from build123d import *

# Parameters (mm, degrees)
SKETCH1_W             = 121.412
SKETCH1_H             = 114.4524
BOSS_EXTRUDE1_DEPTH   = 3.175
FILLET2_R             = 13.97
F_6_CLEARANCE_HOLE1_D = 3.7973


with BuildPart() as part:
    # Sketch1 → Boss-Extrude1 (new body)
    with BuildSketch(Plane(origin=(0, 0, 0), x_dir=(1, 0, 0), z_dir=(0, 1, 0))):
        Rectangle(SKETCH1_W, SKETCH1_H)
    extrude(amount=BOSS_EXTRUDE1_DEPTH)

    # Fillet2
    fillet2_edges = [part.edges().sort_by_distance(p)[0] for p in [
        (-60.706, 1.5875, -57.2262),
        (60.706, 1.5875, -57.2262),
        (60.706, 1.5875, 57.2262),
        (-60.706, 1.5875, 57.2262),
    ]]
    fillet(fillet2_edges, radius=FILLET2_R)

    # #6 Clearance Hole1 (through all)
    with Locations(Plane.XZ):
        with Locations((-25.4, 54.0512), (-25.4, -54.0512), (-57.531, -25.4), (-57.531, 25.4)):
            f_6_clearance_hole1 = Hole(F_6_CLEARANCE_HOLE1_D / 2)

    # Mirror1: #6 Clearance Hole1 across plane
    add(f_6_clearance_hole1.mirror(Plane(origin=(0, 0, 0), x_dir=(0, 0, 1), z_dir=(1, 0, 0))), mode=Mode.SUBTRACT)


solid = part.part
CAD build for the part. Positions are in the model's coordinates, mm. Give positions to 0.01 mm unless a question says otherwise; leave off trailing zeros. Write each loop counter-clockwise with the first axis right and the second up, starting at its lowest first coordinate (ties: lowest second). Pieces come first, ordered by that corner, then holes. Notation, with made-up numbers: (-28.75, 24) - (4.25, 24) arc R18 cw to (4.25, 54) - close; hole circle Ø5 at (60, 33.5). An arc over 180 degrees is marked (long way). Put each result on its own line as item: value.
(1) Wall check: L1, parallel to Z at x = 25.4, y = 1.95; L2, parallel to X at y = 0.6, z = -53; L3, parallel to X at y = 1.7, z = -50.5. Give the ranges that are in metal, low to high.
Working result:
L1: -57.23 to -55.95, -52.15 to 52.15, 55.95 to 57.23
L2: -56.75 to -26.98, -23.82 to 23.82, 26.98 to 56.75
L3: -58.68 to 58.68
(2) Saw through at D-D (z = -50). List the corners of the cut face in (x, y) (3 decimals), then the cut area to 3 significant figures.
Working result:
outline: (-58.97, 0) - (58.97, 0) - (58.97, 3.175) - (-58.97, 3.175) - close
area: 374 mm^2
(3) Saw through at A-A (z = 25.4). List the corners of the cut face in (x, y) (3 decimals), then the cut area to 3 significant figures.
Working result:
outline: (-60.706, 0) - (-59.43, 0) - (-59.43, 3.175) - (-60.706, 3.175) - close; (-55.632, 0) - (55.632, 0) - (55.632, 3.175) - (-55.632, 3.175) - close; (59.43, 0) - (60.706, 0) - (60.706, 3.175) - (59.43, 3.175) - close
area: 361 mm^2
(4) Saw through at C-C (y = 0.9). Count the separate pieces of the cut face and the enclosed holes in it, then the cut area to 3 significant figures.
Working result:
separate pieces: 1
enclosed holes: 8
area: 13,600 mm^2
(5) Saw through at B-B (x = 25.4). List the corners of the cut face in (y, z) (3 decimals), then the cut area to 3 significant figures.
Working result:
outline: (0, -57.226) - (3.175, -57.226) - (3.175, -55.95) - (0, -55.95) - close; (0, -52.153) - (3.175, -52.153) - (3.175, 52.153) - (0, 52.153) - close; (0, 55.95) - (3.175, 55.95) - (3.175, 57.226) - (0, 57.226) - close
area: 339 mm^2
(6) Pull direction Z, two halves, no side cores. Call faces 1 (the cylindrical face through (56.13, 1.61, -24.12)), 2 (the flat face through (-1, 2, -57.226)), 3 (the cylindrical face through (-23.5, 1.6, 54.1)), 4 (the flat face through (-60.706, 2, 1)): released by +Z, released by -Z, zero draft, split by the parting line, or undercut.
Working result:
face 1: undercut
face 2: released by -Z
face 3: undercut
face 4: zero draft
